from build123d import *

# Parameters (mm, degrees)
EXTRUDE_START   = 20.5
SKETCH_1_R      = 1.7
SKETCH_1_W      = 6
SKETCH_1_H      = 8
EXTRUDE_1_DEPTH = 3


with BuildPart() as part:
    # 草圖1 → 填料-伸長1 (new body)
    with BuildSketch(Plane(origin=(0, 0, 0), x_dir=(0, 0, -1), z_dir=(1, 0, 0)).offset(EXTRUDE_START)):
        Polygon((-10.5, 14), (-19.5, 14), (-19.5, 20), (-27.5, 20), (-27.5, 14), (-59.7, 14), (-59.7, 20), (-67.7, 20), (-67.7, 14), (-92, 14), (-92, 20), (-100, 20), (-100, 14), (-131, 14), (-131, 20), (-139, 20), (-139, 14), (-155.5, 14), (-155.5, -14), (-139, -14), (-139, -20), (-131, -20), (-131, -14), (-100, -14), (-100, -20), (-92, -20), (-92, -14), (-67.7, -14), (-67.7, -20), (-59.7, -20), (-59.7, -14), (-27.5, -14), (-27.5, -20), (-19.5, -20), (-19.5, -14), (-10.5, -14), (-10.5, -4), (-16.5, -4), (-16.5, 4), (-10.5, 4), align=None)
        with Locations((-23.5, 17)):
            Circle(SKETCH_1_R, mode=Mode.SUBTRACT)
        with Locations((-23.5, -17)):
            Circle(SKETCH_1_R, mode=Mode.SUBTRACT)
        with Locations((-63.7, 17)):
            Circle(SKETCH_1_R, mode=Mode.SUBTRACT)
        with Locations((-63.7, -17)):
            Circle(SKETCH_1_R, mode=Mode.SUBTRACT)
        with Locations((-96, 17)):
            Circle(SKETCH_1_R, mode=Mode.SUBTRACT)
        with Locations((-96, -17)):
            Circle(SKETCH_1_R, mode=Mode.SUBTRACT)
        with Locations((-135, 17)):
            Circle(SKETCH_1_R, mode=Mode.SUBTRACT)
        with Locations((-135, -17)):
            Circle(SKETCH_1_R, mode=Mode.SUBTRACT)
        with Locations((-86, 0)):
            Rectangle(SKETCH_1_W, SKETCH_1_H, mode=Mode.SUBTRACT)
    extrude(amount=EXTRUDE_1_DEPTH)


solid = part.part
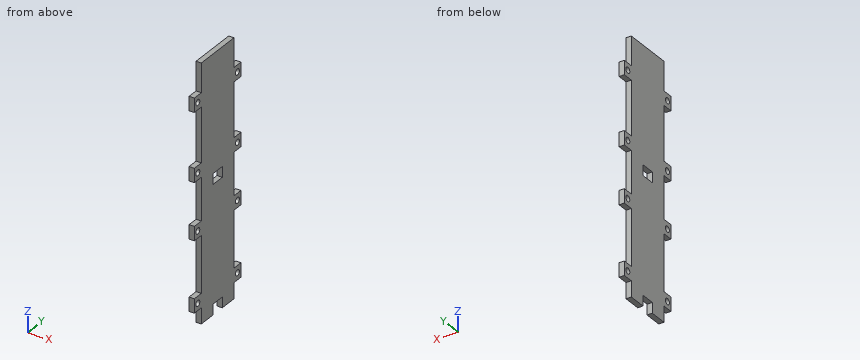
Work out the finished part from the listing and answer in its coordinate system (mm). Round coordinates to 2 decimals unless told otherwise and drop trailing zeros. Write each loop counter-clockwise with the first axis right and the second up, starting at its lowest first coordinate (ties: lowest second). Pieces come first, ordered by that corner, then holes. Notation, with made-up numbers: (77.25, -34.75) -> (120.25, -34.75) arc R19 cw to (120.25, -7.75) -> close; hole circle Ø10 at (-35, 12.5). An arc over 180 degrees is marked (long way). Write each question's results on one line, items separated by ' | '.
Item 1: A cutting plane is placed at B-B, the plane z = 96. Determine the outline of the cut face in (x, y).
Result set:
outline: (20.5, -20) -> (23.5, -20) -> (23.5, -18.7) -> (20.5, -18.7) -> close; (20.5, -15.3) -> (23.5, -15.3) -> (23.5, 15.3) -> (20.5, 15.3) -> close; (20.5, 18.7) -> (23.5, 18.7) -> (23.5, 20) -> (20.5, 20) -> close
Item 2: Find the intervals of material crossed by line 1 along Y through (x, z) = (22.4, 96); line 2 along Y through (x, z) = (22.5, 24.5); line 3 along Y through (x, z) = (23.05, 124), in increasing order. Write a range as [from, to].
Result set:
line 1: [-20, -18.7], [-15.3, 15.3], [18.7, 20] | line 2: [-20, -18.37], [-15.63, 15.63], [18.37, 20] | line 3: [-14, 14]
Item 3: A cutting plane is placed at A-A, the plane y = 0. Determine the outline of the cut face in (x, z), plus the area to 3 significant figures.
Result set:
outline: (20.5, 16.5) -> (23.5, 16.5) -> (23.5, 83) -> (20.5, 83) -> close; (20.5, 89) -> (23.5, 89) -> (23.5, 155.5) -> (20.5, 155.5) -> close | area: 399 mm^2
Item 4: A cutting plane is placed at C-C, the plane y = -17. Count the separate pieces of the cut face and the enclosed holes in it, plus the area to 3 significant figures.
Result set:
separate pieces: 8 | enclosed holes: 0 | area: 55.2 mm^2
Item 5: Flat-ended cylindrical pins translate along their axes: P1, Ø2.5, axis at y = 17, z = 23.5, coming from the +X side; P2, Ø1.5, axis at x = 22, z = 14, coming from the -Y side; P3, Ø4.5, axis at y = -17, z = 23.5, coming from the -X side; P4, Ø0.9, axis at x = 22, z = 111.5, coming from the +Y side. Find the tip coordinate at first contact, or state that the pin passes through.
Result set:
P1: through | P2: y = -14 | P3: x = 20.5 | P4: y = 14
